```python
from build123d import *

# Parameters (mm, degrees)
SKETCH2_W           = 47.625
SKETCH2_H           = 25.4
BOSS_EXTRUDE1_DEPTH = 44.45
SKETCH3_W           = 28.575
SKETCH3_H           = 44.45
CUT_EXTRUDE1_DEPTH  = 26.4
SKETCH4_W           = 40.64
SKETCH4_H           = 19.05
CUT_EXTRUDE2_DEPTH  = 48.625
FILLET1_R           = 2.54
FILLET2_R           = 2.54
SKETCH5_R           = 1.143
CUT_EXTRUDE3_DEPTH  = 45.45
SKETCH6_R           = 1.143
CUT_EXTRUDE4_DEPTH  = 45.45
SKETCH7_R           = 1.143
CUT_EXTRUDE5_DEPTH  = 10.16
SKETCH8_W           = 36.195
SKETCH8_H           = 25.4
CUT_EXTRUDE6_DEPTH  = 26.4
FILLET3_R           = 3.175
FILLET4_R           = 3.175
SKETCH9_W           = 87.912640597
SKETCH9_H           = 53.774742358
CUT_EXTRUDE7_DEPTH  = 35.56


with BuildPart() as part:
    # Sketch2 → Boss-Extrude1 (new body)
    with BuildSketch(Plane.XY):
        Rectangle(SKETCH2_W, SKETCH2_H)
    extrude(amount=BOSS_EXTRUDE1_DEPTH)

    # Sketch3 → Cut-Extrude1 (cut, through all)
    with BuildSketch(Plane(origin=(0, 12.7, 0), x_dir=(1, 0, 0), z_dir=(0, 1, 0))):
        with Locations((0, -22.225)):
            Rectangle(SKETCH3_W, SKETCH3_H)
    extrude(amount=-CUT_EXTRUDE1_DEPTH, mode=Mode.SUBTRACT)

    # Sketch4 → Cut-Extrude2 (cut, through all)
    with BuildSketch(Plane.ZY.offset(23.8125)):
        with Locations((20.32, -3.175)):
            Rectangle(SKETCH4_W, SKETCH4_H)
    extrude(amount=-CUT_EXTRUDE2_DEPTH, mode=Mode.SUBTRACT)

    # Fillet1
    fillet1_edges = [part.edges().sort_by_distance(p)[0] for p in [
        (19.05, 6.35, 40.64),
    ]]
    fillet(fillet1_edges, radius=FILLET1_R)

    # Fillet2
    fillet2_edges = [part.edges().sort_by_distance(p)[0] for p in [
        (-19.05, 6.35, 40.64),
    ]]
    fillet(fillet2_edges, radius=FILLET2_R)

    # Sketch5 → Cut-Extrude3 (cut, through all)
    with BuildSketch(Plane.XY.offset(44.45)):
        with Locations((-19.05, -9.525)):
            Circle(SKETCH5_R)
        with Locations((-19.05, 3.175)):
            Circle(SKETCH5_R)
    extrude(amount=-CUT_EXTRUDE3_DEPTH, mode=Mode.SUBTRACT)

    # Sketch6 → Cut-Extrude4 (cut, through all)
    with BuildSketch(Plane.XY.offset(44.45)):
        with Locations((19.05, -9.525)):
            Circle(SKETCH6_R)
        with Locations((19.05, 3.175)):
            Circle(SKETCH6_R)
    extrude(amount=-CUT_EXTRUDE4_DEPTH, mode=Mode.SUBTRACT)

    # Sketch7 → Cut-Extrude5 (cut)
    with BuildSketch(Plane(origin=(0, 12.7, 0), x_dir=(1, 0, 0), z_dir=(0, 1, 0))):
        with Locations((-17.4625, -38.1)):
            Circle(SKETCH7_R)
        with Locations((17.4625, -38.1)):
            Circle(SKETCH7_R)
        with Locations((-17.4625, -3.175)):
            Circle(SKETCH7_R)
        with Locations((17.4625, -3.175)):
            Circle(SKETCH7_R)
    extrude(amount=-CUT_EXTRUDE5_DEPTH, mode=Mode.SUBTRACT)

    # Sketch8 → Cut-Extrude6 (cut, through all)
    with BuildSketch(Plane(origin=(0, 12.7, 0), x_dir=(1, 0, 0), z_dir=(0, 1, 0))):
        with Locations((0, -20.6375)):
            Rectangle(SKETCH8_W, SKETCH8_H)
    extrude(amount=-CUT_EXTRUDE6_DEPTH, mode=Mode.SUBTRACT)

    # Fillet3
    fillet3_edges = [part.edges().sort_by_distance(p)[0] for p in [
        (-18.0975, 9.525, 33.3375),
        (-18.0975, 9.525, 7.9375),
    ]]
    fillet(fillet3_edges, radius=FILLET3_R)

    # Fillet4
    fillet4_edges = [part.edges().sort_by_distance(p)[0] for p in [
        (18.0975, 9.525, 7.9375),
        (18.0975, 9.525, 33.3375),
    ]]
    fillet(fillet4_edges, radius=FILLET4_R)

    # Sketch9 → Cut-Extrude7 (cut)
    with BuildSketch(Plane(origin=(0, 0, 0), x_dir=(0, 0, -1), z_dir=(1, 0, 0))):
        with Locations((-24.289386177, -0.100701765)):
            Rectangle(SKETCH9_W, SKETCH9_H)
    extrude(amount=CUT_EXTRUDE7_DEPTH, mode=Mode.SUBTRACT)


solid = part.part
```
Model file for the job. Use its own axes, mm. A direction names the side the tool comes from. Coordinates: 2 decimals unless noted, no trailing zeros. Order: outer loops, then holes, each group sorted by start corner. A loop starts at its lowest first (then second) coordinate and runs counter-clockwise, first axis right, second up. Notation, with made-up numbers: M 64.25,-13.5 L 110.25,-13.5 A15 ccw 110.25,-4.5 Z; hole C -30.5,-18.75 d6. An arc over 180 degrees is marked long. Answer as CSV lines item,"result".
(1) Band-saw the part on B-B, the plane y = -10.25. List the corners of the cut face in (x, z).
Geometry says:
outline,"M -23.81,40.64 L -19.93,40.64 L -19.93,44.45 L -23.81,44.45 Z; M -18.17,40.64 L -14.29,40.64 L -14.29,44.45 L -18.17,44.45 Z"
(2) Band-saw the part on D-D, the plane y = 9.25. State how many separate pieces and enclosed holes the cut face has, then the cut area to 3 significant figures.
Geometry says:
separate pieces,"1"
enclosed holes,"2"
area,"323 mm2"
(3) Flat gauge pins, fed straight in: pin 1 (2 mm diameter, centred on y = 3.5, z = 25, fed in from +X); pin 2 (3 mm diameter, centred on x = -19.5, y = -3.5, fed in from -Z); pin 3 (5 mm diameter, centred on x = -20, z = 17.5, fed in from -Y); pin 4 (5 mm diameter, centred on y = 11, z = 20, fed in from +X). Where does each tip first touch, or does it go through?
Geometry says:
pin 1,"passes through"
pin 2,"stops at z = 40.64"
pin 3,"stops at y = 6.35"
pin 4,"stops at x = -18.1"
(4) Band-saw the part on A-A, the plane x = -19.05. List the corners of the cut face in (y, z), then the cut area to 3 significant figures.
Geometry says:
outline,"M -12.7,40.64 L -10.67,40.64 L -10.67,44.45 L -12.7,44.45 Z; M -8.38,40.64 L 2.03,40.64 L 2.03,44.45 L -8.38,44.45 Z; M 4.32,40.59 A2.54 cw 6.35,38.1 L 6.35,0 L 12.7,0 L 12.7,44.45 L 4.32,44.45 Z"
area,"339 mm2"
(5) 3-axis set-ups, long thin cutter, end or side, ignore diameter. For faces 4 (the cylindrical face through (-17.143, 9.481, 32.432)), 5 (the flat face through (-20, 6.35, 19)), 6 (the cylindrical face through (-17.96, 3.52, 42.55)): which of +Z, -Z, +X, -X, +Y, -Y reach the whole face in a straight line?
Geometry says:
face 4,"+X, +Y, -Y"
face 5,"-Z, +X, -X, -Y"
face 6,"+Z, -Z"
(6) Pull direction Y, two halves, no side cores. Call faces 1 (the flat face through (-23.812, 7, 27)), 2 (the cylindrical face through (-17.96, -9.18, 42.57)), 3 (the flat face through (-20, 12.7, 22)): +Y half, -Y half, draft (parallel to the pull), parting line (faces both ways), or undercut.
Geometry says:
face 1,"draft"
face 2,"undercut"
face 3,"+Y half"
(7) Wall check: line 1 along Y through (x, z) = (-19.05, 42.75); line 2 along Y through (x, z) = (-22.5, 8.5); line 3 along Z through (x, y) = (-17, 0). Give the ranges that are in metal, low to high.
Geometry says:
line 1,"y = -12.7 to -10.67, -8.38 to 2.03, 4.32 to 12.7"
line 2,"y = 6.35 to 12.7"
line 3,"z = 40.64 to 44.45"
(8) Band-saw the part on C-C, the plane x = -21.75. List the corners of the cut face in (y, z).
Geometry says:
outline,"M -12.7,40.64 L 3.81,40.64 A2.54 cw 6.35,38.1 L 6.35,0 L 12.7,0 L 12.7,44.45 L -12.7,44.45 Z"
